Job drawing, mm, ordinate dimensions from the low corner. One solid piece. A direction names the side the tool comes from. Give positions to 0.01 mm unless a question says otherwise; leave off trailing zeros. Loops run counter-clockwise (first coordinate to the right, second up) from the corner with the lowest first, then second, coordinate; pieces in that order, holes last. Notation, with made-up numbers: (83, 16) -> (92, 16) arc R28 ccw to (92, 49) -> close; hole circle Ø4 at (39, 81). An arc over 180 degrees is marked (long way). Answer as a JSON object with one key per item and string values. Group by question number.
Q1. Band-saw the part on C-C, the plane y = 52. Write the cut outline in (x, z).
Q2. Drop flat-ended pins along their axis: pin 1 (1.5 mm diameter, centred on x = 7, y = 26, fed in from -Z); pin 2 (0.8 mm diameter, centred on x = 9.5, y = 1, fed in from -Z). Give the stop position or say it passes through.
Q3. Band-saw the part on B-B, the plane y = 70. Write the cut outline in (x, z).
Q4. Tool access for the marked faces 4 and 5: list every direction of +Z, -Z, +X, -X, +Y, -Y with a clear straight run to the whole face (end or side of a thin tool).
Q5. Wall check: probe 1 along Z at (x, y) = (23.75, 70.5); probe 2 along Y at (x, z) = (12, 9) (1 decimal); probe 3 along Y at (x, z) = (19.75, 12.5) (1 decimal). Give the ranges that are in metal, low to high. Write a range as from..to.
Q6. Two-plate mould, pull along Y, no slides. Class the marked faces 1, 2 and 3: pulls with the +Y half, pulls with the -Y half, needs draft (parallel to the pull), parting line crosses it, or undercut.
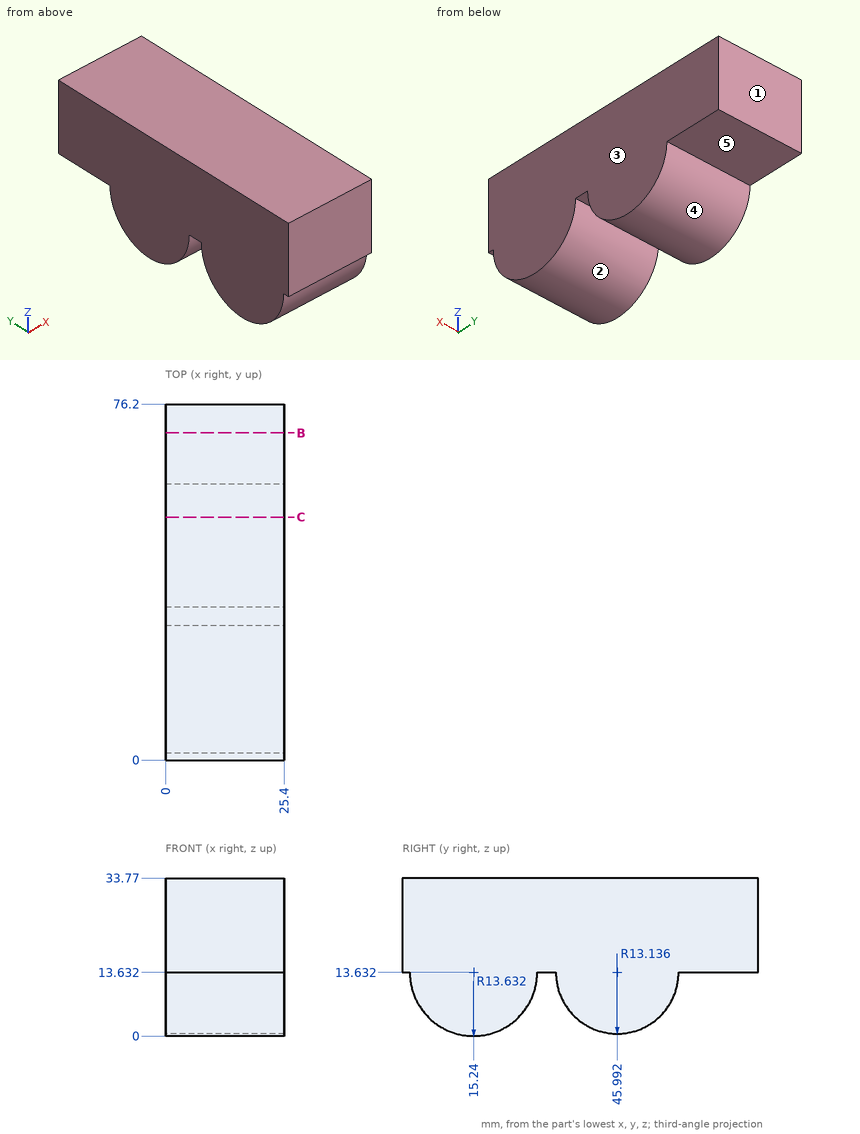
Worked answers:
{
 "1": {"outline": "(0, 1.95) -> (25.4, 1.95) -> (25.4, 33.77) -> (0, 33.77) -> close"},
 "2": {"pin 1": "z = 4.38", "pin 2": "z = 13.63"},
 "3": {"outline": "(0, 13.63) -> (25.4, 13.63) -> (25.4, 33.77) -> (0, 33.77) -> close"},
 "4": {"face 4": "-Z, +X, -X", "face 5": "-Z, +X, -X, +Y"},
 "5": {"probe 1": "13.63..33.77", "probe 2": "2.4..28.1, 33.7..58.3", "probe 3": "1.7..28.8, 32.9..59.1"},
 "6": {"face 1": "pulls with the +Y half", "face 2": "undercut", "face 3": "needs draft"}
}
